Part model, mm, in its own coordinate system. A direction names the side the tool comes from. Round coordinates to 2 decimals unless told otherwise and drop trailing zeros. Loops run counter-clockwise (first coordinate to the right, second up) from the corner with the lowest first, then second, coordinate; pieces in that order, holes last. Notation, with made-up numbers: (61.25, 77.25) - (96.25, 77.25) arc R12 cw to (96.25, 93.25) - close; hole circle Ø8 at (25.5, 6.25). An arc over 180 degrees is marked (long way). Put each result on its own line as item: value.
Autodesk Inventor part; units mm, degrees
ref_plane "WorkPlane2" through (0, 0, 0) normal (0, 0, 1) x (1, 0, 0)
ref_plane "Work Plane2" through (0, 0, -3.15) normal (0, 0, 1) x (1, 0, 0)
ref_plane "WorkPlane3" through (0, 0, 7) normal (0, 0, 1) x (1, 0, 0)
ref_plane "WorkPlane2" through (0, 0, 0) normal (0, 0, 1) x (1, 0, 0)
sketch "Sketch1" plane through (0, 0, 0) normal (1, 0, 0) x (0, 1, 0)
  point P0 (0, 0)
ref_plane "Work Plane2" through (0, 0, -3.15) normal (0, 0, 1) x (1, 0, 0)
ref_plane "WorkPlane3" through (0, 0, 7) normal (0, 0, 1) x (1, 0, 0)
sketch "Sketch2" plane through (0, 0, 0) normal (0, 1, 0) x (-1, 0, 0)
  point P0 (0, 0)
sketch "Sketch3" plane through (0, 0, 0) normal (1, 0, 0) x (0, 1, 0)
  line L0 (1.75, -4.35) -> (1.45, -3.75)
  line L1 (1.75, -5.8) -> (1.75, -4.35)
  line L2 (0, -5.8) -> (1.75, -5.8)
  line L3 (0, 0) -> (0, -5.8)
  arc A0 (3.65, -0.8) -> (0, 0) centre (0, -8.7266) ccw
  line L4 (3.65, -0.95) -> (3.65, -0.8)
  line L5 (1.45, -3.15) -> (3.65, -0.95)
  line L6 (1.45, -3.75) -> (1.45, -3.15)
  line L7 (0, -31.6445) -> (0, 31.6445) construction
  line L8 (0, -31.6445) -> (0, 31.6445)
  line L9 (0, -44.3023) -> (0, 44.3023)
  dimension "d2" = 1.75
  dimension "d4" = 1.45
  dimension "d6" = 0.6
  dimension "d8" = 2.35
  dimension "d10" = 135
  dimension "d12" = 3.65
  dimension "d14" = 0
  dimension "d16" = 0.8
  dimension "d18" = 5
  dimension "d22" = 1.45
revolve "Revolution1" add sketch "Sketch3" angle 360 about axis through (0, 0, -31.6445) along (0, 0, 1)
fillet "Fillet1" radius 0.9 1 edges at (0, -1.45, -3.15)
sketch "Sketch4" plane through (0, 0, 0) normal (0, 1, 0) x (-1, 0, 0)
  line L0 (0, 0) -> (-2.4, 0)
  line L1 (0, -2) -> (0, 0)
  line L2 (-2.4, 0) -> (-0.4, -2)
  line L3 (0, -10.4719) -> (0, 1.7453)
  arc A0 (3.65, -0.8) -> (-3.65, -0.8) centre (0, -8.7266) ccw
  line L4 (0, -2) -> (-0.4, -2)
  point P0 (0, -2.4)
  dimension "d30" = 45
  dimension "d33" = 4.8
  dimension "d34" = 0.4
  dimension "d35" = 90
extrude "Extrusion1" cut sketch "Sketch4" along normal mid plane 0.8
pattern_circular "PolarArray1" count 4 over 360 about axis through (0, 0, -10) along (0, 0, 1) of "Extrusion1"
thread "Thread1"
ref_plane "MSC_PF1" through (0, 0, 0) normal (1, 0, 0) x (0, 1, 0)
ref_plane "MSC_PT1" through (0, 3.65, -0.95) normal (0, 0, -1) x (-1, 0, 0)
equation "\"d2\" = 0.5 * NND"
equation "\"d4\" = 0.5 * msp_mdtds"
equation "\"d6\" = msp_x"
equation "\"d8\" = ParK"
equation "\"d12\" = 0.5 * Dk"
equation "\"d16\" = ParF"
equation "\"d18\" = NLG"
equation "\"d22\" = b"
equation "\"d24\" = r"
equation "\"d33\" = M"
equation "\"d31\" = 0.166667 * M"
equation "\"d39\" = b"
equation "\"PTC\" = 0.6"
equation "\"msp_x\" = PTC"
equation "\"NLG\" = 5"
equation "\"NND\" = 3.5"
equation "\"ParK\" = 2.35"
equation "\"r\" = 0.9"
equation "\"msp_mdtds\" = NND - PTC"
equation "\"b\" = 1.45"
equation "\"Dk\" = 7.3"
equation "\"ParF\" = 0.8"
equation "\"M\" = 4.8"
equation "\"ParA\" = 1.2"
equation "\"THREADDIA\" = NND"
equation "\"TEMPLATE\" = 1.2345"
properties part number "ISO 7047 - M3.5x5 - 4.8 - H" material "Steel"
1. Band-saw the part on A-A (z = -1.05). List the corners of the cut face in (x, y).
A:
outline: circle Ø7.1 at (0, 0); hole (-1.35, -0.4) - (-0.4, -0.4) - (-0.4, -1.35) - (0.4, -1.35) - (0.4, -0.4) - (1.35, -0.4) - (1.35, 0.4) - (0.4, 0.4) - (0.4, 1.35) - (-0.4, 1.35) - (-0.4, 0.4) - (-1.35, 0.4) - close
2. Tool access for faces 4 (the cylindrical face through (0.67, 1.617, -5.065)), 5 (the flat face through (-1, 0.4, -1)): list every direction of +Z, -Z, +X, -X, +Y, -Y with a clear straight run to the whole face (end or side of a thin tool).
A:
face 4: -Z
face 5: +Z
3. Two-plate mould, pull along X, no slides. Class faces 1 (the conical face through (1.791, -0.398, -2.765)), 2 (the flat face through (0, 0, -5.8)), 3 (the flat face through (0.4, -1, -1)): pulls with the +X half, pulls with the -X half, needs draft (parallel to the pull), parting line crosses it, or undercut.
A:
face 1: parting line crosses it
face 2: needs draft
face 3: undercut
4. Probe line 1 along Y through (x, z) = (-1.25, -0.75); line 2 along Y through (x, z) = (0.25, -0.7); line 3 along Z through (x, y) = (-2.5, 1). List the from-to ranges inside material, lowest first. Write a range as [from, to].
A:
line 1: y = [-3.31, -0.4], [0.4, 3.31]
line 2: y = [-3.42, -1.7], [1.7, 3.42]
line 3: z = [-1.91, -0.43]
5. Band-saw the part on B-B (z = -5.05). List the corners of the cut face in (x, y).
A:
outline: circle Ø3.5 at (0, 0)
6. Pin check, flat tips, straight feed: P1, Ø1.9, axis at x = 1.5, z = -1.5, coming from the +Y side; P2, Ø3, axis at x = 0.5, z = -3.5, coming from the +Y side; P3, Ø0.5, axis at y = -1.5, z = -1.5, coming from the +X side; P4, Ø2, axis at y = -1, z = -1, coming from the +X side. Stop position of each tip, or through.
A:
P1: stops at y = 3.58
P2: stops at y = 2.57
P3: stops at x = 3.02
P4: stops at x = 3.65
7. Band-saw the part on C-C (z = -2.5). List the corners of the cut face in (x, y).
A:
outline: circle Ø4.2 at (0, 0)
